Source: CAD feature listing. Evaluate the final solid. Frame: model axes, mm. Coordinates: 2 decimals unless noted, no trailing zeros. Order: outer loops, then holes, each group sorted by start corner. A loop starts at its lowest first (then second) coordinate and runs counter-clockwise, first axis right, second up. Notation, with made-up numbers: (-34.5, 0.25) -> (-7.5, 0.25) arc R31 cw to (-7.5, 39.25) -> close; hole circle Ø7 at (59.25, 89). An arc over 180 degrees is marked (long way). Write item = value, one per line. Start each with the question number.
Item 1: Ray query, line 1 along Z through (x, y) = (59.5, 6.25); line 2 along X through (y, z) = (1, -2); line 3 along Z through (x, y) = (33.5, 1.5). Return the intervals inside material, ascending. Write a range as [from, to].
Item 2: Section query C-C (x = 20). Output: boundary loops of the cut face in (y, z).
Item 3: Section query A-A (y = 5). Count the separate pieces of the cut face and the enclosed holes in it, then the cut area to 3 significant figures.
Item 4: Contact query for flat-ended pins moving along their axis: pin 1 (5 mm diameter, centred on x = 45.96, z = 0, fed in from -Y); pin 2 (2.5 mm diameter, centred on x = 58.66, z = 0, fed in from -Y); pin 3 (1 mm diameter, centred on x = 73, y = 5, fed in from +Z); pin 4 (1 mm diameter, centred on y = 1, z = -2.5, fed in from -X). Output: stop coordinate, or through.
Item 5: Section query B-B (x = 40). Output: boundary loops of the cut face in (y, z) (3 decimals).
Item 6: Mould query, pull axis X, two halves, no side actions, for faces 1 (the cylindrical face through (85.53, 3.22, 0.61)), 2 (the cylindrical face through (100.246, 3.219, -3.356)). Classes: released by +X, released by -X, zero draft, split by the parting line, or undercut.
```python
from build123d import *

# Parameters (mm, degrees)
BOSS_EXTRUDE1_DEPTH = 6.35
FILLET1_R           = 4.837495
FILLET3_R           = 6.251556
SKETCH3_R           = 3.175
SKETCH3_R_2         = 1.5875
CUT_EXTRUDE1_DEPTH  = 7.35
SKETCH5_R           = 1.5875
CUT_EXTRUDE2_DEPTH  = 7.35
LPATTERN1_COUNT     = 11
LPATTERN1_PITCH     = 6.35


with BuildPart() as part:
    # Sketch2 → Boss-Extrude1 (new body)
    with BuildSketch(Plane(origin=(0, 0, 0), x_dir=(1, 0, 0), z_dir=(0, 1, 0))):
        Polygon((0, 0), (0, 6.35), (101.6, 4.7625), (101.6, 0), align=None)
    boss_extrude1 = extrude(amount=BOSS_EXTRUDE1_DEPTH)

    # Mirror1: Boss-Extrude1 across plane
    add(boss_extrude1.mirror(Plane(origin=(101.6, 6.35, 0), x_dir=(1, 0, 0), z_dir=(0, 0, -1))))

    # Fillet1
    fillet1_edges = [part.edges().sort_by_distance(p)[0] for p in [
        (101.6, 3.175, 4.7625),
        (101.6, 3.175, -4.7625),
    ]]
    fillet(fillet1_edges, radius=FILLET1_R)

    # Fillet3
    fillet3_edges = [part.edges().sort_by_distance(p)[0] for p in [
        (0, 3.175, 6.35),
        (0, 3.175, -6.35),
    ]]
    fillet(fillet3_edges, radius=FILLET3_R)

    # Sketch3 → Cut-Extrude1 (cut, through all)
    with BuildSketch(Plane(origin=(0, 6.35, 0), x_dir=(1, 0, 0), z_dir=(0, 1, 0))):
        with Locations((6.251556349, 0)):
            Circle(SKETCH3_R)
        with Locations((96.762504613, 0)):
            Circle(SKETCH3_R_2)
    extrude(amount=-CUT_EXTRUDE1_DEPTH, mode=Mode.SUBTRACT)

    # Sketch5 → Cut-Extrude2 (cut, through all)
    with BuildSketch(Plane(origin=(0, 6.35, 0), x_dir=(1, 0, 0), z_dir=(0, 1, 0))):
        with Locations((90.412504613, 0)):
            Circle(SKETCH5_R)
    cut_extrude2 = extrude(amount=-CUT_EXTRUDE2_DEPTH, mode=Mode.SUBTRACT)

    # LPattern1: Cut-Extrude2 ×11
    with Locations(*[(-i * LPATTERN1_PITCH, 0, 0) for i in range(1, LPATTERN1_COUNT)]):
        add(cut_extrude2, mode=Mode.SUBTRACT)


solid = part.part
```
Computed:
q1.line_1 = [-5.42, -1.35], [1.35, 5.42]
q1.line_2 = [0.33, 3.79], [8.72, 101.17]
q1.line_3 = [-5.83, -1.57], [1.57, 5.83]
q2.outline = (0, -6.04) -> (6.35, -6.04) -> (6.35, 6.04) -> (0, 6.04) -> close
q3.separate_pieces = 1
q3.enclosed_holes = 13
q3.area = 975 mm^2
q4.pin_1 = 0
q4.pin_2 = through
q4.pin_3 = 5.22
q4.pin_4 = 0.33
q5.outline = (0, -5.725) -> (6.35, -5.725) -> (6.35, -1.539) -> (0, -1.539) -> close; (0, 1.539) -> (6.35, 1.539) -> (6.35, 5.725) -> (0, 5.725) -> close
q6.face_1 = undercut
q6.face_2 = released by +X
